Verification items for the finished model (mm, model axes). Coordinates: 2 decimals unless noted, no trailing zeros. Write each loop counter-clockwise with the first axis right and the second up, starting at its lowest first coordinate (ties: lowest second). Pieces come first, ordered by that corner, then holes. Notation, with made-up numbers: (12, 55.25) -> (20, 55.25) arc R19 cw to (20, 87.25) -> close; hole circle Ø8 at (70, -18.75). An arc over 180 degrees is marked (long way). Answer in a Markdown table with one row per item.
```python
from build123d import *

# Parameters (mm, degrees)
SKETCH1_R           = 0.5
SKETCH1_R_2         = 0.25
BOSS_EXTRUDE2_DEPTH = 0.3
SKETCH2_R           = 0.15
CUT_EXTRUDE1_DEPTH  = 10
CIRPATTERN2_COUNT   = 4
SKETCH3_R           = 0.15
CUT_EXTRUDE2_DEPTH  = 10
CIRPATTERN3_COUNT   = 4


with BuildPart() as part:
    # Sketch1 → Boss-Extrude2 (new body)
    with BuildSketch(Plane.XY):
        with BuildLine():
            Line((0, 0), (0, 9.6))
            ThreePointArc((0, 9.6), (1.25, 10.85), (2.5, 9.6))
            Line((2.5, 9.6), (2.5, 0))
            ThreePointArc((2.5, 0), (1.25, -1.25), (0, 0))
        make_face()
        with Locations((1.25, 9.6)):
            Circle(SKETCH1_R, mode=Mode.SUBTRACT)
        with Locations((1.25, 0)):
            Circle(SKETCH1_R, mode=Mode.SUBTRACT)
        with Locations((0.5, 4.8)):
            Circle(SKETCH1_R_2, mode=Mode.SUBTRACT)
        with Locations((2, 4.8)):
            Circle(SKETCH1_R_2, mode=Mode.SUBTRACT)
    extrude(amount=BOSS_EXTRUDE2_DEPTH)

    # Sketch2 → Cut-Extrude1 (cut)
    with BuildSketch(Plane.XY.offset(0.3)):
        with Locations((0.25, 9.6)):
            Circle(SKETCH2_R)
    cut_extrude1 = extrude(amount=-CUT_EXTRUDE1_DEPTH, mode=Mode.SUBTRACT)

    # CirPattern2: Cut-Extrude1 ×4 about axis
    cirpattern2_axis = Axis((1.25, 9.6, 0), (0, 0, 1))
    for i in range(1, CIRPATTERN2_COUNT):
        add(cut_extrude1.rotate(cirpattern2_axis, i * 360 / CIRPATTERN2_COUNT), mode=Mode.SUBTRACT)

    # Sketch3 → Cut-Extrude2 (cut)
    with BuildSketch(Plane.XY.offset(0.3)):
        with Locations((2.25, 0)):
            Circle(SKETCH3_R)
    cut_extrude2 = extrude(amount=-CUT_EXTRUDE2_DEPTH, mode=Mode.SUBTRACT)

    # CirPattern3: Cut-Extrude2 ×4 about axis
    cirpattern3_axis = Axis((1.25, 0, 0), (0, 0, 1))
    for i in range(1, CIRPATTERN3_COUNT):
        add(cut_extrude2.rotate(cirpattern3_axis, i * 360 / CIRPATTERN3_COUNT), mode=Mode.SUBTRACT)


solid = part.part
```
1. Thickness scan on line 1 (Y direction, x = 1.55, z = 0.1); line 2 (Y direction, x = 1.05, z = 0.25); line 3 (X direction, y = -1, z = 0.2). Record the ranges inside material, lowest first. Write a range as from..to.
Geometry says:
| item | result |
|---|---|
| line 1 | -1.21..-0.4, 0.4..9.2, 10..10.81 |
| line 2 | -1.23..-0.46, 0.46..9.14, 10.06..10.83 |
| line 3 | 0.5..1.1, 1.4..2 |
2. Section check B-B, the plane x = 1.25. Record the boundary of the cut face in (y, z), plus the area to 3 significant figures.
Geometry says:
| item | result |
|---|---|
| outline | (-1.25, 0) -> (-1.15, 0) -> (-1.15, 0.3) -> (-1.25, 0.3) -> close; (-0.85, 0) -> (-0.5, 0) -> (-0.5, 0.3) -> (-0.85, 0.3) -> close; (0.5, 0) -> (0.85, 0) -> (0.85, 0.3) -> (0.5, 0.3) -> close; (1.15, 0) -> (8.45, 0) -> (8.45, 0.3) -> (1.15, 0.3) -> close; (8.75, 0) -> (9.1, 0) -> (9.1, 0.3) -> (8.75, 0.3) -> close; (10.1, 0) -> (10.45, 0) -> (10.45, 0.3) -> (10.1, 0.3) -> close; (10.75, 0) -> (10.85, 0) -> (10.85, 0.3) -> (10.75, 0.3) -> close |
| area | 2.67 mm^2 |
3. Section check C-C, the plane x = 0.5. Record the boundary of the cut face in (y, z), plus the area to 3 significant figures.
Geometry says:
| item | result |
|---|---|
| outline | (-1, 0) -> (4.55, 0) -> (4.55, 0.3) -> (-1, 0.3) -> close; (5.05, 0) -> (10.6, 0) -> (10.6, 0.3) -> (5.05, 0.3) -> close |
| area | 3.33 mm^2 |
4. Section check D-D, the plane y = 4.8. Record the boundary of the cut face in (x, z).
Geometry says:
| item | result |
|---|---|
| outline | (0, 0) -> (0.25, 0) -> (0.25, 0.3) -> (0, 0.3) -> close; (0.75, 0) -> (1.75, 0) -> (1.75, 0.3) -> (0.75, 0.3) -> close; (2.25, 0) -> (2.5, 0) -> (2.5, 0.3) -> (2.25, 0.3) -> close |
5. Section check A-A, the plane y = 8.6. Record the boundary of the cut face in (x, z).
Geometry says:
| item | result |
|---|---|
| outline | (0, 0) -> (1.1, 0) -> (1.1, 0.3) -> (0, 0.3) -> close; (1.4, 0) -> (2.5, 0) -> (2.5, 0.3) -> (1.4, 0.3) -> close |
